The listing builds one solid part. Answer for the finished solid, in the listing's coordinates (mm). A direction names the side the tool comes from. Give positions to 0.01 mm unless a question says otherwise; leave off trailing zeros. Order: outer loops, then holes, each group sorted by start corner. A loop starts at its lowest first (then second) coordinate and runs counter-clockwise, first axis right, second up. Notation, with made-up numbers: (-37.75, 82.5) - (-20.75, 82.5) arc R25 cw to (-20.75, 118.5) - close; hole circle Ø5 at (44.25, 27). An arc over 180 degrees is marked (long way). Answer in a Markdown table with one row per item.
from build123d import *

# Parameters (mm, degrees)
F0_W     = 95.5
F0_H     = 105.5
F0_W_2   = 22
F0_H_2   = 22
F0_W_3   = 92.5
F0_H_3   = 32
F1_DEPTH = 50
F2_W     = 95.5
F2_H     = 105.5
F3_DEPTH = 1.5
F5_DEPTH = 100
F6_R     = 2
F7_R     = 1


with BuildPart() as f1:
    # F0 (on Top) → F1 (new body)
    with BuildSketch(Plane.XY):
        with Locations((46.25, 51.25)):
            Rectangle(F0_W, F0_H)
        with Locations((11, 11)):
            Rectangle(F0_W_2, F0_H_2, mode=Mode.SUBTRACT)
        with Locations((34.5, 11)):
            Rectangle(F0_W_2, F0_H_2, mode=Mode.SUBTRACT)
        with Locations((11, 34.5)):
            Rectangle(F0_W_2, F0_H_2, mode=Mode.SUBTRACT)
        with Locations((34.5, 34.5)):
            Rectangle(F0_W_2, F0_H_2, mode=Mode.SUBTRACT)
        with Locations((58, 11)):
            Rectangle(F0_W_2, F0_H_2, mode=Mode.SUBTRACT)
        with Locations((81.5, 11)):
            Rectangle(F0_W_2, F0_H_2, mode=Mode.SUBTRACT)
        with Locations((58, 34.5)):
            Rectangle(F0_W_2, F0_H_2, mode=Mode.SUBTRACT)
        with Locations((81.5, 34.5)):
            Rectangle(F0_W_2, F0_H_2, mode=Mode.SUBTRACT)
        with Locations((11, 91.5)):
            Rectangle(F0_W_2, F0_H_2, mode=Mode.SUBTRACT)
        with Locations((34.5, 91.5)):
            Rectangle(F0_W_2, F0_H_2, mode=Mode.SUBTRACT)
        with Locations((46.25, 63)):
            Rectangle(F0_W_3, F0_H_3, mode=Mode.SUBTRACT)
        with Locations((58, 91.5)):
            Rectangle(F0_W_2, F0_H_2, mode=Mode.SUBTRACT)
        with Locations((81.5, 91.5)):
            Rectangle(F0_W_2, F0_H_2, mode=Mode.SUBTRACT)
    extrude(amount=F1_DEPTH)

    # F2 (on Top) → F3 (join)
    with BuildSketch(Plane.XY):
        with Locations((46.25, 51.25)):
            Rectangle(F2_W, F2_H)
    extrude(amount=F3_DEPTH)

    # F4 (on face) → F5 (cut)
    with BuildSketch(Plane(origin=(-1.5, 0, 0), x_dir=(0, -1, 0), z_dir=(-1, 0, 0))):
        with BuildLine():
            Line((1.5, 50), (-79, 50))
            add(Edge.make_bspline(
                [(-79, 50), (-70.9814525391, 39.139632946), (-62.9629050781, 28.2792658921), (-51.25, 25)],
                knots=[0, 0, 0, 0, 0.4547652437, 0.4547652437, 0.4547652437, 0.4547652437], degree=3))
            add(Edge.make_bspline(
                [(-51.25, 25), (-37.2069678319, 21.0683676592), (-17.853483916, 28.0341838296), (1.5, 35)],
                knots=[0.4547652437, 0.4547652437, 0.4547652437, 0.4547652437, 1, 1, 1, 1], degree=3))
            Line((1.5, 35), (1.5, 50))
        make_face()
    extrude(amount=-F5_DEPTH, mode=Mode.SUBTRACT)

    # F6
    f6_edges = [f1.edges().sort_by_distance(p)[0] for p in [
        (94, -1.5, 17.5),
        (94, 104, 25),
        (-1.5, -1.5, 17.5),
        (-1.5, 104, 25),
    ]]
    fillet(f6_edges, radius=F6_R)

    # F7
    f7_edges = [f1.edges().sort_by_distance(p)[0] for p in [
        (0, 0, 17.980133),
        (92.5, 0, 17.980133),
        (92.5, 102.5, 25.75),
        (0, 102.5, 25.75),
    ]]
    fillet(f7_edges, radius=F7_R)


solid = f1.part
Item 1: Each of these flat-tipped pins is pushed along its axis until it touches: P1, Ø6, axis at x = 22.5, y = 65.5, coming from the +Z side; P2, Ø17.5, axis at x = 6.5, y = 91.5, coming from the +Z side. Where does it stop, or does it pass through?
Answer block:
| item | result |
|---|---|
| P1 | z = 1.5 |
| P2 | z = 50 |
Item 2: Determine the mould class of faces 1 (the face through (94, 62, 19)), 2 (the face through (47, 11, 18)), 3 (the face through (46, -1.5, 17)) for opening direction Y: pulls with the +Y half, pulls with the -Y half, needs draft (parallel to the pull), parting line crosses it, or undercut.
Answer block:
| item | result |
|---|---|
| face 1 | needs draft |
| face 2 | undercut |
| face 3 | pulls with the -Y half |
Item 3: Find section B-B on z = 6.5. Count the separate pieces of the cut face and the enclosed holes in it, then the cut area to 3 significant figures.
Answer block:
| item | result |
|---|---|
| separate pieces | 1 |
| enclosed holes | 13 |
| area | 1,300 mm² |
Item 4: Find section A-A on y = 85.5. Write down the section's boundary in (x, z).
Answer block:
| item | result |
|---|---|
| outline | (-1.5, 0) - (94, 0) - (94, 50) - (92.5, 50) - (92.5, 1.5) - (70.5, 1.5) - (70.5, 50) - (69, 50) - (69, 1.5) - (47, 1.5) - (47, 50) - (45.5, 50) - (45.5, 1.5) - (23.5, 1.5) - (23.5, 50) - (22, 50) - (22, 1.5) - (0, 1.5) - (0, 50) - (-1.5, 50) - close |
Item 5: Consider line 1 (Y direction, x = 36, z = 4); line 2 (X direction, y = 13.5, z = 9.5); line 3 (Y direction, x = 63, z = 24.5). Determine where each line is inside the solid, lowest interval first.
Answer block:
| item | result |
|---|---|
| line 1 | -1.5 to 0, 22 to 23.5, 45.5 to 47, 79 to 80.5, 102.5 to 104 |
| line 2 | -1.5 to 0, 22 to 23.5, 45.5 to 47, 69 to 70.5, 92.5 to 94 |
| line 3 | -1.5 to 0, 22 to 23.5, 79 to 80.5, 102.5 to 104 |
Item 6: Which of the six approach directions +Z, -Z, +X, -X, +Y, -Y give full straight-line access (tool end or side, diameter ignored) to faces 4 (the face through (92.5, 11, 18)), 5 (the face through (46, 91, 50))?
Answer block:
| item | result |
|---|---|
| face 4 | +Z |
| face 5 | +Z, +X, -X, +Y, -Y |
